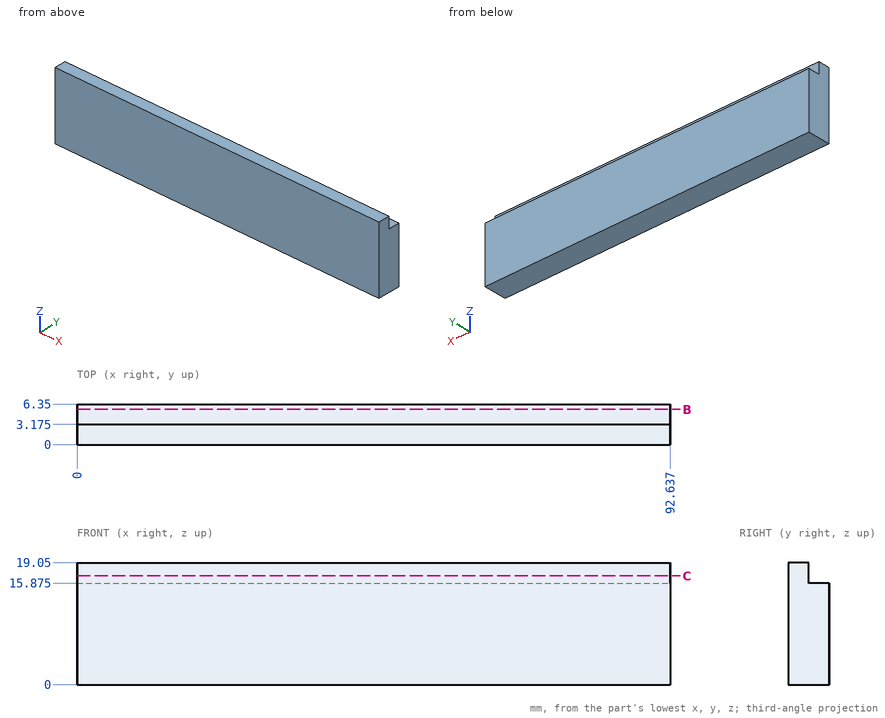
Part print with two shaded views. Sizes in mm from the minimum x, y, z corner. Round coordinates to 2 decimals unless told otherwise and drop trailing zeros. Order: outer loops, then holes, each group sorted by start corner. A loop starts at its lowest first (then second) coordinate and runs counter-clockwise, first axis right, second up. Notation, with made-up numbers: (82.5, -13.75) -> (128.5, -13.75) arc R19 ccw to (128.5, 13.25) -> close; hole circle Ø6 at (35, 17). An arc over 180 degrees is marked (long way). One line per question, with ' | ' between items.
Q1. Slice it at C-C (z = 17). Write the cut outline in (x, y) (1 decimal), then the cut area to 3 significant figures.
Completed:
outline: (0, 0) -> (92.6, 0) -> (92.6, 3.2) -> (0, 3.2) -> close | area: 294 mm^2
Q2. Probe probe 1 along Y at (x, z) = (42, 18) (1 decimal); probe 2 along Z at (x, y) = (61, 5) (1 decimal). List the from-to ranges inside material, lowest first.
Completed:
probe 1: y = 0 to 3.2 | probe 2: z = 0 to 15.9
Q3. Slice it at B-B (y = 5.5). Write the cut outline in (x, z) (1 decimal).
Completed:
outline: (0, 0) -> (92.6, 0) -> (92.6, 15.9) -> (0, 15.9) -> close
Q4. Drop flat-ended pins along their axis: pin 1 (4 mm diameter, centred on x = 72.5, z = 14, fed in from -Y); pin 2 (1 mm diameter, centred on x = 54, z = 17.5, fed in from +Y) (1 decimal); pin 3 (1.6 mm diameter, centred on x = 37.5, y = 4.5, fed in from +Z) (1 decimal). Give the stop position or say it passes through.
Completed:
pin 1: stops at y = 0 | pin 2: stops at y = 3.2 | pin 3: stops at z = 15.9
